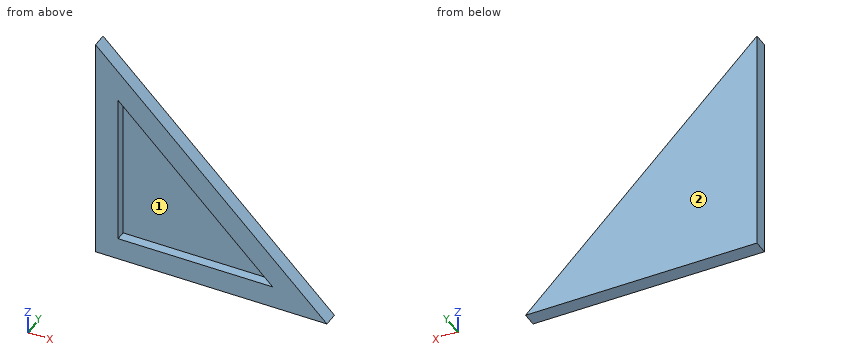
```python
from build123d import *

# Parameters (mm, degrees)
F0_R     = 9.525
F1_DEPTH = 38.1
F2_DEPTH = 19.05


with BuildPart() as f1:
    # F0 (on Front) → F1 (new body)
    with BuildSketch(Plane.XZ):
        Polygon((914.4, 0), (0, 914.4), (0, 0), align=None)
        with Locations((44.45, 44.45)):
            Circle(F0_R, mode=Mode.SUBTRACT)
        Polygon((699.776414305, 88.9), (88.9, 88.9), (88.9, 699.776414305), align=None, mode=Mode.SUBTRACT)
        with Locations((44.45, 44.45)):
            Circle(F0_R)
    extrude(amount=F1_DEPTH)

    # F0 (on Front) → F2 (join)
    with BuildSketch(Plane.XZ):
        Polygon((914.4, 0), (0, 914.4), (0, 0), align=None)
        with Locations((44.45, 44.45)):
            Circle(F0_R, mode=Mode.SUBTRACT)
        Polygon((699.776414305, 88.9), (88.9, 88.9), (88.9, 699.776414305), align=None, mode=Mode.SUBTRACT)
        Polygon((88.9, 699.776414305), (88.9, 88.9), (699.776414305, 88.9), align=None)
        with Locations((44.45, 44.45)):
            Circle(F0_R)
    extrude(amount=-F2_DEPTH)


solid = f1.part
```
Here's how the part is built. I have some questions about the finished solid (model axes, mm). Face numbers are marked on the shaded views. Coordinates: 2 decimals unless noted, no trailing zeros. Write each loop counter-clockwise with the first axis right and the second up, starting at its lowest first coordinate (ties: lowest second). Pieces come first, ordered by that corner, then holes. Notation, with made-up numbers: M 81,11 L 129,11 A12 cw 129,32 Z; hole C 0,-12.5 d6. An arc over 180 degrees is marked long. Answer as CSV lines item,"result". Start each with the question number.
Q1. Suppose I cut it at A-A, the plane y = -19. List the corners of the cut face in (x, z) for me.
Q2. Will these pins go through, and if not, where does the flat tip stop? pin 1 Ø19 at (y, z) = (-23, 371.5) entering from +X; pin 2 Ø3 at (x, z) = (120.5, 438.5) entering from -Y; pin 3 Ø19 at (x, y) = (259, -14) entering from +Z.
Q3. If we mould it in two halves opening along X, with no side actions, what happens to the marked faces 1 and 2? For each: pulls with the +X half, pulls with the -X half, needs draft (parallel to the pull), parting line crosses it, or undercut.
Q4. Suppose I cut it at C-C, the plane x = 138.5. List the corners of the cut face in (y, z) for me.
Q5. I need wall thicknesses on probe 1 along Y at (x, z) = (95.5, 279.5); probe 2 along X at (y, z) = (-3, 527.5); probe 3 along Z at (x, y) = (545, -33). Which ranges of each line are inside material? Lowest first, please. Write a range as [from, to].
Q6. Suppose I cut it at B-B, the plane z = 427. List the corners of the cut face in (x, y) for me, then the cut area to 3 significant figures.
Q7. Suppose I cut it at D-D, the plane x = 720. List the corners of the cut face in (y, z) for me, then the cut area to 3 significant figures.
Entries:
1,outline,"M 0,0 L 914.4,0 L 0,914.4 Z; hole M 88.9,88.9 L 699.78,88.9 L 88.9,699.78 Z"
2,pin 1,"stops at x = 552.4"
2,pin 2,"stops at y = 0"
2,pin 3,"stops at z = 664.9"
3,face 1,"undercut"
3,face 2,"needs draft"
4,outline,"M -38.1,0 L 19.05,0 L 19.05,775.9 L -38.1,775.9 L -38.1,650.18 L 0,650.18 L 0,88.9 L -38.1,88.9 Z"
5,probe 1,"y = [0, 19.05]"
5,probe 2,"x = [0, 88.9], [261.18, 386.9]"
5,probe 3,"z = [0, 88.9], [243.68, 369.4]"
6,outline,"M 0,-38.1 L 88.9,-38.1 L 88.9,0 L 361.68,0 L 361.68,-38.1 L 487.4,-38.1 L 487.4,19.05 L 0,19.05 Z"
6,area,"17,500 mm²"
7,outline,"M -38.1,0 L 19.05,0 L 19.05,194.4 L -38.1,194.4 Z"
7,area,"11,100 mm²"
